from build123d import *

# Parameters (mm, degrees)
SZKIC2_R                    = 5
DODANIE_WYCI_GNI_CIE1_DEPTH = 270


with BuildPart() as part:
    # Szkic1 → Obrót1 (revolve)
    with BuildSketch(Plane.XY):
        with BuildLine():
            Line((0, 8), (0, -8))
            ThreePointArc((0, -8), (8, 0), (0, 8))
        make_face()
    revolve(axis=Axis((0, 8, 0), (0, -1, 0)))

    # Szkic2 → Dodanie-wyciągnięcie1 (add)
    with BuildSketch(Plane(origin=(0, 0, 0), x_dir=(1, 0, 0), z_dir=(0, 1, 0))):
        with Locations(Location((0, 0, 0), (0, 0, 90))):
            Circle(SZKIC2_R)
    extrude(amount=DODANIE_WYCI_GNI_CIE1_DEPTH)

    # Szkic3 → Obrót2 (revolve)
    with BuildSketch(Plane.XY):
        with BuildLine():
            Line((0, 270), (-15.5, 270))
            ThreePointArc((-15.5, 270), (-18.681980515, 268.681980515), (-20, 265.5))
            Line((-20, 265.5), (-20, 174.5))
            ThreePointArc((-20, 174.5), (-18.681980515, 171.318019485), (-15.5, 170))
            Line((-15.5, 170), (-12.25, 170))
            ThreePointArc((-12.25, 170), (-9.068019485, 168.681980515), (-7.75, 165.5))
            Line((-7.75, 165.5), (-7.75, 144.5))
            ThreePointArc((-7.75, 144.5), (-6.431980515, 141.318019485), (-3.25, 140))
            Line((-3.25, 140), (0, 140))
            Line((0, 140), (0, 270))
        make_face()
    revolve(axis=Axis((0, 270, 0), (0, -1, 0)))


solid = part.part
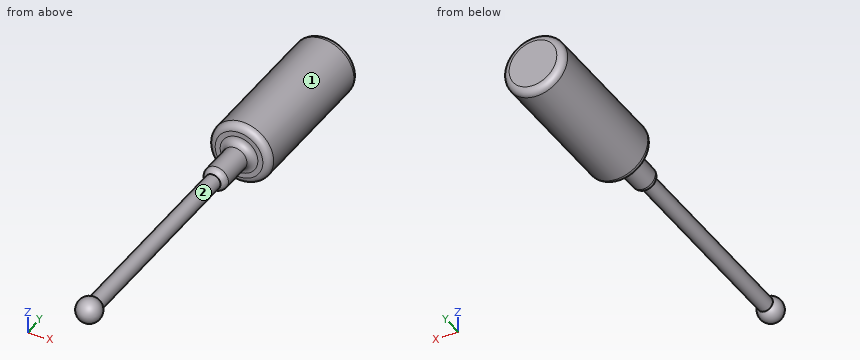
Work out the finished part from the listing and answer in its coordinate system (mm). Face numbers are marked on the shaded views. A direction names the side the tool comes from. Give positions to 0.01 mm unless a question says otherwise; leave off trailing zeros. Loops run counter-clockwise (first coordinate to the right, second up) from the corner with the lowest first, then second, coordinate; pieces in that order, holes last. Notation, with made-up numbers: (-28.5, 20.25) -> (14.5, 20.25) arc R11 ccw to (14.5, 25.25) -> close; hole circle Ø2 at (5.25, 21.5). An arc over 180 degrees is marked (long way). Use a Markdown table: item, result. Add a question column.
1) The part is cut by section A-A, the plane y = 15.5. Determine the outline of the cut face in (x, z).
2) Consider line 1 along Y through (x, z) = (-6, -4.5); line 2 along Y through (x, z) = (-1, -15.5); line 3 along Z through (x, y) = (-16, 222). Determine where each line is inside the solid, lowest interval first.
3) Each of these flat-tipped pins is pushed along its axis until it touches: P1, Ø6, axis at x = 2.5, y = 94, coming from the -Z side; P2, Ø8, axis at x = -2.5, y = 227, coming from the +Z side; P3, Ø12, axis at y = 134.5, z = 2, coming from the +X side. Where does it stop, or does it pass through?
4) The part is cut by section B-B, the plane y = 251. Determine the outline of the cut face in (x, z).
5) Which of the six approach directions +Z, -Z, +X, -X, +Y, -Y give full straight-line access (tool end or side, diameter ignored) to the marked faces 1 and 2?
Reported:
| question | item | result |
|---|---|---|
| 1 | outline | circle Ø10 at (0, 0) |
| 2 | line 1 | y = -2.78 to 2.78, 143.02 to 270 |
| 2 | line 2 | y = 170 to 270 |
| 2 | line 3 | z = -12 to 12 |
| 3 | P1 | stops at z = -5 |
| 3 | P2 | stops at z = 20 |
| 3 | P3 | stops at x = 5.07 |
| 4 | outline | circle Ø40 at (0, 0) |
| 5 | face 1 | +Y, -Y |
| 5 | face 2 | none |
